from build123d import *

# Parameters (mm, degrees)
BOSS_EXTRUDE1_DEPTH = 4.5
SKETCH2_R           = 5.85
BOSS_EXTRUDE2_DEPTH = 0.5
SKETCH3_R           = 4
BOSS_EXTRUDE3_DEPTH = 35


with BuildPart() as part:
    # Sketch1 → Boss-Extrude1 (new body)
    with BuildSketch(Plane.XY):
        Polygon((-6.411545587, -3.901975976), (0.173437527, -7.503549344), (6.584983114, -3.601573368), (6.411545587, 3.901975976), (-0.173437527, 7.503549344), (-6.584983114, 3.601573368), align=None)
    extrude(amount=BOSS_EXTRUDE1_DEPTH)

    # Sketch2 → Boss-Extrude2 (add)
    with BuildSketch(Plane.XY.offset(4.5)):
        Circle(SKETCH2_R)
    extrude(amount=BOSS_EXTRUDE2_DEPTH)

    # Sketch3 → Boss-Extrude3 (add)
    with BuildSketch(Plane.XY.offset(5)):
        Circle(SKETCH3_R)
    extrude(amount=BOSS_EXTRUDE3_DEPTH)


solid = part.part
Build history of the part. All positions in model axes, mm. A direction names the side the tool comes from. Give positions to 0.01 mm unless a question says otherwise; leave off trailing zeros. Order: outer loops, then holes, each group sorted by start corner. A loop starts at its lowest first (then second) coordinate and runs counter-clockwise, first axis right, second up. Notation, with made-up numbers: M 37,80.25 L 86,80.25 A22 cw 86,94.25 Z; hole C 32,-25.5 d2. An arc over 180 degrees is marked long. Use one line per item in the form item = value.
1) Probe probe 1 along Z at (x, y) = (0.5, -4); probe 2 along Z at (x, y) = (4.5, -4); probe 3 along X at (y, z) = (-4.75, 4). List the from-to ranges inside material, lowest first.
Calculated:
probe_1 = 0 to 5
probe_2 = 0 to 4.5
probe_3 = -4.86 to 4.7
2) Saw through at B-B (y = 0). Give the cut face in (x, z).
Calculated:
outline = M -6.5,0 L 6.5,0 L 6.5,4.5 L 5.85,4.5 L 5.85,5 L 4,5 L 4,40 L -4,40 L -4,5 L -5.85,5 L -5.85,4.5 L -6.5,4.5 Z
3) Drop flat-ended pins along their axis: pin 1 (6 mm diameter, centred on x = 4.5, z = 5.5, fed in from -Y); pin 2 (1 mm diameter, centred on x = -1, z = 14, fed in from +Y); pin 3 (6 mm diameter, centred on x = -1, z = 12, fed in from -Y). Give the stop position or say it passes through.
Calculated:
pin_1 = -6.59
pin_2 = 3.97
pin_3 = -4
4) Tool access for faces 1 (the face through (0, 0, 40)), 2 (the face through (-1.27, -5.71, 4.75)): list every direction of +Z, -Z, +X, -X, +Y, -Y with a clear straight run to the whole face (end or side of a thin tool).
Calculated:
face_1 = +Z, +X, -X, +Y, -Y
face_2 = +Z
5) Saw through at A-A (x = -4.75). Give the cut face in (y, z), plus the area to 3 significant figures.
Calculated:
outline = M -4.81,0 L 4.72,0 L 4.72,4.5 L 3.41,4.5 L 3.41,5 L -3.41,5 L -3.41,4.5 L -4.81,4.5 Z
area = 46.3 mm2
6) Saw through at D-D (x = -2.75). Give the cut face in (y, z).
Calculated:
outline = M -5.9,0 L 5.94,0 L 5.94,4.5 L 5.16,4.5 L 5.16,5 L 2.9,5 L 2.9,40 L -2.9,40 L -2.9,5 L -5.16,5 L -5.16,4.5 L -5.9,4.5 Z
7) Saw through at C-C (z = 12.5). Give the cut face in (x, y).
Calculated:
outline = C 0,0 d8
